```python
from build123d import *

# Parameters (mm, degrees)
F1_R      = 7.5
F3_R      = 12.5
F4_DEPTH  = 12.5
F5_R      = 6
F6_DEPTH  = 25
F9_DEPTH  = 12.5
F10_R     = 6
F11_DEPTH = 25


with BuildPart() as f2:
    # F2: sweep along a path in F0
    with BuildLine(Plane.XY) as f2_path:
        Line((150, -12), (125, -12))
        ThreePointArc((125, -12), (81.789999989, -9.4166667579), (39.1955835962, -1.7034700315))
        ThreePointArc((39.1955835962, -1.7034700315), (32.1487132371, -0.4273896908), (25, 0))
        Line((25, 0), (0, 0))
    # F1 (on Right) → F2 (sweep)
    with BuildSketch(Plane.YZ):
        Circle(F1_R)
    sweep(path=f2_path.line)

    # F3 (on Front) → F4 (join, symmetric)
    with BuildSketch(Plane.XZ):
        Circle(F3_R)
    extrude(amount=F4_DEPTH, both=True)

    # F5 (on face) → F6 (cut)
    with BuildSketch(Plane.XZ.offset(12.5)):
        Circle(F5_R)
    extrude(amount=-F6_DEPTH, mode=Mode.SUBTRACT)

    # F8 (on offset) → F9 (join, symmetric)
    with BuildSketch(Plane.XZ.offset(12)):
        with BuildLine():
            Line((140, -7.5), (150, -7.5))
            Line((150, -7.5), (150, 7.5))
            Line((150, 7.5), (140, 7.5))
            ThreePointArc((140, 7.5), (137.5, 0), (140, -7.5))
        make_face()
        with BuildLine():
            Line((150, 7.5), (150, -7.5))
            Line((150, -7.5), (140, -7.5))
            ThreePointArc((140, -7.5), (153.9528470752, -11.8585412256), (162.5, 0))
            ThreePointArc((162.5, 0), (153.9528470752, 11.8585412256), (140, 7.5))
            Line((140, 7.5), (150, 7.5))
        make_face()
    extrude(amount=F9_DEPTH, both=True)

    # F10 (on face) → F11 (cut)
    with BuildSketch(Plane.XZ.offset(24.5)):
        with Locations((150, 0)):
            Circle(F10_R)
    extrude(amount=-F11_DEPTH, mode=Mode.SUBTRACT)


solid = f2.part
```
Geometry: final body of the model. Coordinates: model frame, mm. A direction names the side the tool comes from. Round coordinates to 2 decimals unless told otherwise and drop trailing zeros. Order: outer loops, then holes, each group sorted by start corner. A loop starts at its lowest first (then second) coordinate and runs counter-clockwise, first axis right, second up. Notation, with made-up numbers: (-26, -37.5) -> (-10, -37.5) arc R24 ccw to (-10, -3.5) -> close; hole circle Ø3 at (56.25, 78). An arc over 180 degrees is marked (long way). Use one line per item in the form item = value. Start each with the question number.
1. Cut plane C-C (x = 22). Return the cut outline in (y, z), then the cut area to 3 significant figures.
2. Cut plane A-A (x = 0). Return the cut outline in (y, z).
3. Line query: probe 1 along Z at (x, y) = (0, -1); probe 2 along X at (y, z) = (10, -0.5); probe 3 along Y at (x, z) = (-4, 7). Output: solid intervals per line, ascending.
4. Cut plane B-B (z = 4.5). Return the cut outline in (x, y).
5. Draft query along Z for faces 1 (the face through (-3, 12.5, -5.4)), 2 (the face through (17.4, 6.93, 2.87)), 3 (the face through (145.24, -12.18, -3.65)). Return one class per face: pulls with the +Z half, pulls with the -Z half, needs draft (parallel to the pull), parting line crosses it, or undercut.
6. Reachability of faces 4 (the face through (-3, -12.5, -5.4)), 5 (the face through (147, -24.5, -5.4)), 6 (the face through (-6, 0, 0)), 7 (the face through (147, 0.5, -5.4)), 8 (the face through (132.395, -4.846, -2.253)) from +Z, -Z, +X, -X, +Y, -Y: full face, straight path, thin tool, end or side. Return the list, or none.
7. Pin query (flat end, axial travel): pin 1 Ø3 at (y, z) = (-11, 2.5) entering from +X; pin 2 Ø2 at (y, z) = (-8.5, 3) entering from +X; pin 3 Ø12.5 at (x, z) = (153, -3.5) entering from +Y. Return the tip coordinate at first contact, or that it passes through.
Solution:
q1.outline = circle Ø15 at (0, 0)
q1.area = 177 mm^2
q2.outline = (-12.5, -12.5) -> (12.5, -12.5) -> (12.5, -6) -> (-12.5, -6) -> close; (-12.5, 6) -> (12.5, 6) -> (12.5, 12.5) -> (-12.5, 12.5) -> close
q3.probe_1 = -12.5 to -6, 6 to 12.5
q3.probe_2 = -12.49 to -5.98, 5.98 to 12.49
q3.probe_3 = -12.5 to 12.5
q4.outline = (-11.66, -12.5) -> (-3.97, -12.5) -> (-3.97, 12.5) -> (-11.66, 12.5) -> close; (3.97, -12.5) -> (11.66, -12.5) -> (11.66, -6) -> (25, -6) arc R54 cw to (37.78, -7.53) arc R368.67 ccw to (125, -18) -> (138.34, -18) -> (138.34, -24.5) -> (146.03, -24.5) -> (146.03, 0.5) -> (138.34, 0.5) -> (138.34, -6) -> (125, -6) arc R356.67 cw to (40.62, 4.13) arc R66 ccw to (25, 6) -> (11.66, 6) -> (11.66, 12.5) -> (3.97, 12.5) -> close; (153.97, -24.5) -> (161.66, -24.5) -> (161.66, 0.5) -> (153.97, 0.5) -> close
q5.face_1 = needs draft
q5.face_2 = parting line crosses it
q5.face_3 = undercut
q6.face_4 = +Z, -Z, -X, -Y
q6.face_5 = +Z, -Z, +X, -X, -Y
q6.face_6 = +Y, -Y
q6.face_7 = +Z, -Z, +X, +Y
q6.face_8 = none
q7.pin_1 = 162.46
q7.pin_2 = 162.34
q7.pin_3 = 0.5
